For this review, use the dimensioned drawing (mm, ordinates from the lowest corner) and the shaded views. A direction names the side the tool comes from. Give positions to 0.01 mm unless a question says otherwise; leave off trailing zeros. Loops run counter-clockwise (first coordinate to the right, second up) from the corner with the lowest first, then second, coordinate; pieces in that order, holes last. Notation, with made-up numbers: M 79.5,-9.75 L 107.5,-9.75 A21 ccw 107.5,1.25 Z; hole C 65.5,44.25 d9. An arc over 180 degrees is marked long. Use a Markdown table: item, result. Add a question column.
(1) Add section A-A, the plane y = 30.5. Give the boundary of the cut face in (x, z) (1 decimal).
(2) For probe 1 along X at (y, z) = (39.5, 0.95) (1 decimal); probe 2 along Y at (x, z) = (30, 1.95) (1 decimal); probe 3 along X at (y, z) = (38, 4.7) (1 decimal), list the stretches that pass through material, from the lowest coordinate up.
(3) Add section D-D, the plane x = 5. Give the boundary of the cut face in (y, z) (1 decimal).
(4) Insertion check: pin 1 Ø1.5 at (y, z) = (15.5, 2.5) entering from -X (1 decimal); pin 2 Ø1.5 at (x, z) = (41.5, 2.5) entering from -Y; pin 3 Ø8.5 at (x, y) = (11.5, 17.5) entering from +Z; pin 4 Ø3 at (y, z) = (6.5, 3) entering from -X (1 decimal). Each pin has a flat end and moves straight along its axis. Give the tip position at first contact, or say it passes through.
(5) Add section B-B, the plane x = 22. Give the boundary of the cut face in (y, z) (1 decimal), then the cut area to 3 significant figures.
(6) For the marked faces 1, 2, 3, 4 and 5, list the 3-axis set-ups (+Z, -Z, +X, -X, +Y, -Y) from which the entire face can be reached by the end or side of a thin tool; tool diameter is ignored.
(7) Add section C-C, the plane y = 40. Give the boundary of the cut face in (x, z), then the cut area to 3 significant figures.
(8) Draft analysis for pull direction X (two halves, no side actions). For the marked faces 6, 7 and 8, state which applies: pulls with the +X half, pulls with the -X half, needs draft (parallel to the pull), parting line crosses it, or undercut.
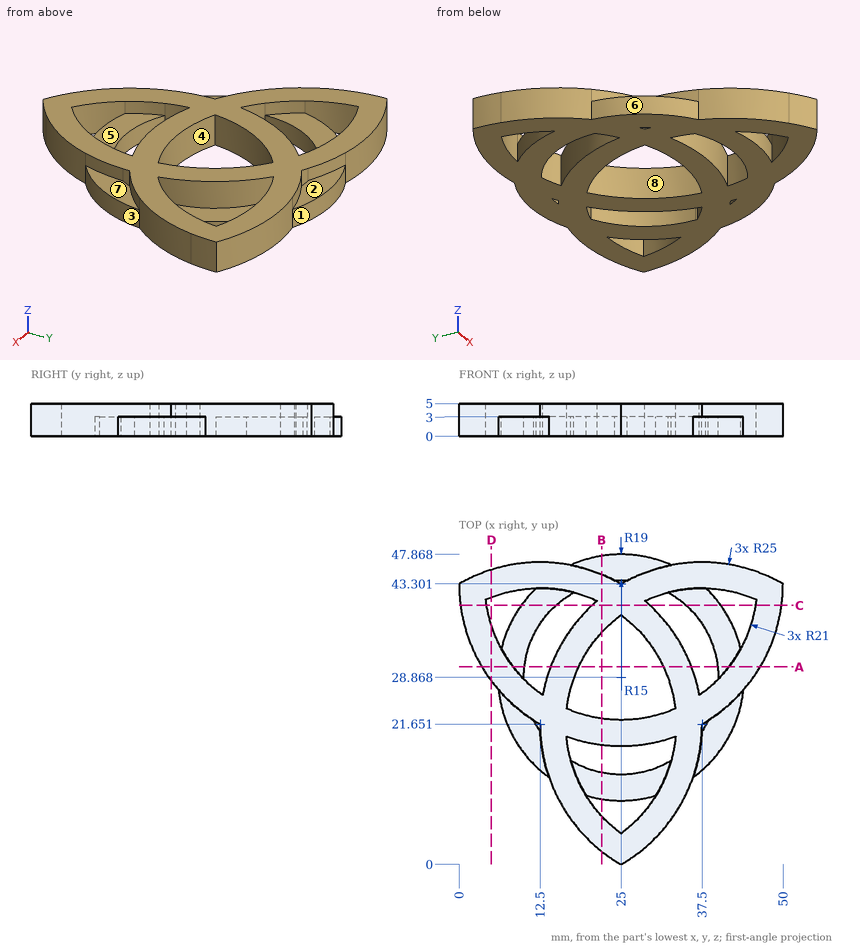
Established:
| question | item | result |
|---|---|---|
| 1 | outline | M 3.5,0 L 10.1,0 L 10.1,3 L 8.4,3 L 8.4,5 L 3.5,5 Z; M 14.1,0 L 18.5,0 L 18.5,5 L 14.1,5 Z; M 31.5,0 L 35.9,0 L 35.9,5 L 31.5,5 Z; M 39.9,0 L 46.5,0 L 46.5,5 L 41.6,5 L 41.6,3 L 39.9,3 Z |
| 2 | probe 1 | 0.3 to 4.3, 9.3 to 14.4, 20 to 30, 35.6 to 40.7, 45.7 to 49.7 |
| 2 | probe 2 | 3.8 to 10, 10.5 to 14.7, 18.8 to 22.9, 33.3 to 39.5, 41.3 to 47.2 |
| 2 | probe 3 | 0.6 to 4.7, 18.6 to 24.3, 25.7 to 31.4, 45.3 to 49.4 |
| 3 | outline | M 28.3,0 L 36.9,0 L 36.9,5 L 28.3,5 Z; M 41.3,0 L 45.5,0 L 45.5,5 L 41.3,5 Z |
| 4 | pin 1 | x = 10.8 |
| 4 | pin 2 | y = 18.24 |
| 4 | pin 3 | z = 5 |
| 4 | pin 4 | x = 16.6 |
| 5 | outline | M 2,0 L 7.5,0 L 7.5,5 L 2,5 Z; M 10.1,0 L 14.2,0 L 14.2,3 L 10.1,3 Z; M 18.5,0 L 22.5,0 L 22.5,5 L 18.5,5 Z; M 35.8,0 L 47.6,0 L 47.6,3 L 44.8,3 L 44.8,5 L 35.8,5 Z |
| 5 | area | 113 mm^2 |
| 6 | face 1 | +Z, -Z, +Y |
| 6 | face 2 | +Z, +Y |
| 6 | face 3 | +Z, -Z, +X, -Y |
| 6 | face 4 | +Z, -Z |
| 6 | face 5 | +Z |
| 7 | outline | M 0.22,0 L 4.26,0 L 4.26,5 L 0.22,5 Z; M 9.6,0 L 14.95,0 L 14.95,3 L 9.6,3 Z; M 20.52,0 L 29.48,0 L 29.48,5 L 20.52,5 Z; M 35.05,0 L 40.4,0 L 40.4,3 L 35.05,3 Z; M 45.74,0 L 49.78,0 L 49.78,5 L 45.74,5 Z |
| 7 | area | 117 mm^2 |
| 8 | face 6 | pulls with the -X half |
| 8 | face 7 | needs draft |
| 8 | face 8 | undercut |
